from build123d import *

# Parameters (mm, degrees)
F2_DEPTH  = 25.4
F3_R      = 28.575
F4_DEPTH  = 63.5
F5_R      = 15.875
F6_DEPTH  = 57.15
F9_R      = 6.35
F10_DEPTH = 63.5
F11_R     = 3.175
F12_DEPTH = 25.4


with BuildPart() as f2:
    # F1 (on face) → F2 (new body)
    with BuildSketch(Plane.XZ):
        Polygon((5.08, 135.130365), (5.08, 206.777484), (0, 217.17), (-5.08, 206.777484), (-5.08, 135.130365), (-23.009013, 85.870806), (0, 0), (23.009013, 85.870806), align=None)
        Polygon((63.165773, 119.566329), (23.009013, 85.870806), (0, 0), (62.861793, 62.861793), (71.964591, 114.486329), (107.788151, 176.534554), (108.585, 188.074737), (98.989333, 181.614554), align=None)
        Polygon((-62.861793, 62.861793), (0, 0), (-23.009013, 85.870806), (-63.165773, 119.566329), (-98.989333, 181.614554), (-108.585, 188.074737), (-107.788151, 176.534554), (-71.964591, 114.486329), align=None)
        Polygon((-85.870806, 23.009013), (0, 0), (-62.861793, 62.861793), (-114.486329, 71.964591), (-176.534554, 107.788151), (-188.074737, 108.585), (-181.614554, 98.989333), (-119.566329, 63.165773), align=None)
        Polygon((-85.870806, -23.009013), (0, 0), (-85.870806, 23.009013), (-135.130365, 5.08), (-206.777484, 5.08), (-217.17, 0), (-206.777484, -5.08), (-135.130365, -5.08), align=None)
        Polygon((-62.861793, -62.861793), (0, 0), (-85.870806, -23.009013), (-119.566329, -63.165773), (-181.614554, -98.989333), (-188.074737, -108.585), (-176.534554, -107.788151), (-114.486329, -71.964591), align=None)
        Polygon((-23.009013, -85.870806), (0, 0), (-62.861793, -62.861793), (-71.964591, -114.486329), (-107.788151, -176.534554), (-108.585, -188.074737), (-98.989333, -181.614554), (-63.165773, -119.566329), align=None)
        Polygon((23.009013, -85.870806), (0, 0), (-23.009013, -85.870806), (-5.08, -135.130365), (-5.08, -206.777484), (0, -217.17), (5.08, -206.777484), (5.08, -135.130365), align=None)
        Polygon((62.861793, -62.861793), (0, 0), (23.009013, -85.870806), (63.165773, -119.566329), (98.989333, -181.614554), (108.585, -188.074737), (107.788151, -176.534554), (71.964591, -114.486329), align=None)
        Polygon((85.870806, -23.009013), (0, 0), (62.861793, -62.861793), (114.486329, -71.964591), (176.534554, -107.788151), (188.074737, -108.585), (181.614554, -98.989333), (119.566329, -63.165773), align=None)
        Polygon((85.870806, 23.009013), (0, 0), (85.870806, -23.009013), (135.130365, -5.08), (206.777484, -5.08), (217.17, 0), (206.777484, 5.08), (135.130365, 5.08), align=None)
        Polygon((62.861793, 62.861793), (0, 0), (85.870806, 23.009013), (119.566329, 63.165773), (181.614554, 98.989333), (188.074737, 108.585), (176.534554, 107.788151), (114.486329, 71.964591), align=None)
    extrude(amount=F2_DEPTH)

    # F3 (on face) → F4 (join)
    with BuildSketch(Plane.XZ):
        Circle(F3_R)
    extrude(amount=F4_DEPTH)

    # F5 (on face) → F6 (cut)
    with BuildSketch(Plane.XZ):
        Circle(F5_R)
    extrude(amount=F6_DEPTH, mode=Mode.SUBTRACT)

    # F9 (on offset) → F10 (cut)
    with BuildSketch(Plane.XY.offset(28.575)):
        with Locations((0, -44.45)):
            Circle(F9_R)
    extrude(amount=-F10_DEPTH, mode=Mode.SUBTRACT)

    # F11 (on face) → F12 (cut)
    with BuildSketch(Plane.XZ):
        with Locations((0, -88.9)):
            Circle(F11_R)
        with Locations((0, 88.9)):
            Circle(F11_R)
    extrude(amount=F12_DEPTH, mode=Mode.SUBTRACT)


solid = f2.part
Check sheet for the modelled part. Datum: model origin and axes. Units: mm. A direction names the side the tool comes from. Give positions to 0.01 mm unless a question says otherwise; leave off trailing zeros. Write each loop counter-clockwise with the first axis right and the second up, starting at its lowest first coordinate (ties: lowest second). Pieces come first, ordered by that corner, then holes. Notation, with made-up numbers: (28, 77.5) -> (51, 77.5) arc R27 ccw to (51, 115.5) -> close; hole circle Ø1 at (-17, 61). An arc over 180 degrees is marked (long way). One line per item, written item: value. Start each with the question number.
Item 1: Section check C-C on z = -158. Record the cut outline in (x, y), then the cut area to 3 significant figures.
Item 2: Section check A-A on y = -44.45. Record the cut outline in (x, z) (3 decimals).
Item 3: Gauge pin test, flat ends, axial feed: pin 1 (10 mm diameter, centred on x = 0, y = -44.45, fed in from -Z); pin 2 (7.5 mm diameter, centred on x = 163, y = -11.5, fed in from -Z); pin 3 (20.5 mm diameter, centred on y = -13, z = 188.5, fed in from -X) (3 decimals); pin 4 (7.5 mm diameter, centred on x = -173, y = -18, fed in from -Z). Record the tip position at first contact, or that the pin passes through.
Item 4: Section check B-B on x = 79. Record the cut outline in (y, z).
Item 5: Tool access check on faces 4 (the flat face through (151.025, -12.522, -81.328)), 5 (the flat face through (13.919, -12.522, -110.845)), 6 (the flat face through (-170, -13, 5.08)), 7 (the cylindrical face through (13.19, -44.18, -25.35)), 8 (the cylindrical face through (14.664, -28.175, -6.08)). Record the directions out of +Z, -Z, +X, -X, +Y, -Y that give a thin tool (end or side, any length) a straight path to the whole face; none if there is none.
Item 6: Draft check along X on faces 1 (the flat face through (-171, -13, -5.08)), 2 (the flat face through (5.08, -13, 170)), 3 (the flat face through (-108.18, -12.52, -182.22)). Enter one of: +X half, -X half, draft (parallel to the pull), parting line (faces both ways), or undercut.
Item 7: Material ranges on probe 1 along Z at (x, y) = (0, -15) (3 decimals); probe 2 along Y at (x, z) = (0, 19); probe 3 along Z at (x, y) = (0, -36.5) (3 decimals), recorded low to high. Write a range as from..to.
Item 8: Section check D-D on y = -15. State how many separate pieces and enclosed holes the cut face has, then the cut area to 3 significant figures.
Results list:
1. outline: (-97.09, -25.4) -> (-85.36, -25.4) -> (-85.36, 0) -> (-97.09, 0) -> close; (-5.08, -25.4) -> (5.08, -25.4) -> (5.08, 0) -> (-5.08, 0) -> close; (85.36, -25.4) -> (97.09, -25.4) -> (97.09, 0) -> (85.36, 0) -> close
1. area: 854 mm²
2. outline: (-6.35, -27.861) -> (-6.35, -14.55) arc R15.875 cw to (-6.35, 14.55) -> (-6.35, 27.861) arc R28.575 ccw to start; (6.35, -27.861) arc R28.575 ccw to (6.35, 27.861) -> (6.35, 14.55) arc R15.875 cw to (6.35, -14.55) -> close
3. pin 1: through
3. pin 2: z = -102.14
3. pin 3: x = -108.585
3. pin 4: z = -107.8
4. outline: (-25.4, -146.99) -> (0, -146.99) -> (0, -126.67) -> (-25.4, -126.67) -> close; (-25.4, -65.71) -> (0, -65.71) -> (0, 65.71) -> (-25.4, 65.71) -> close; (-25.4, 126.67) -> (0, 126.67) -> (0, 146.99) -> (-25.4, 146.99) -> close
5. face 4: +X, +Y, -Y
5. face 5: -Z, +Y, -Y
5. face 6: -X, +Y, -Y
5. face 7: -Y
5. face 8: +Y
6. face 1: draft
6. face 2: undercut
6. face 3: -X half
7. probe 1: -217.17..-92.075, -85.725..-15.875, 15.875..85.725, 92.075..217.17
7. probe 2: -63.5..-50.8, -38.1..0
7. probe 3: -28.575..-15.875, 15.875..28.575
8. separate pieces: 1
8. enclosed holes: 3
8. area: 48,800 mm²
